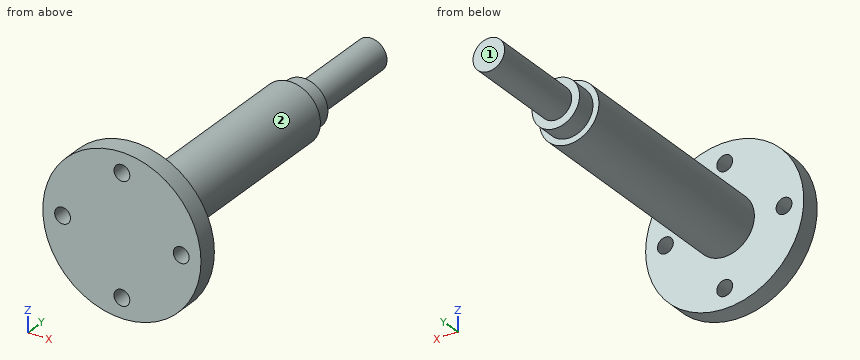
from build123d import *

# Parameters (mm, degrees)
SKETCH1_R           = 20
BOSS_EXTRUDE1_DEPTH = 5
SKETCH2_R           = 7.5
BOSS_EXTRUDE2_DEPTH = 63
SKETCH3_R           = 4
BOSS_EXTRUDE3_DEPTH = 25
SKETCH4_R           = 2
CUT_EXTRUDE1_DEPTH  = 25
SKETCH5_R           = 7.5
SKETCH5_R_2         = 6
CUT_EXTRUDE2_DEPTH  = 5


with BuildPart() as part:
    # Sketch1 → Boss-Extrude1 (new body)
    with BuildSketch(Plane(origin=(0, 0, 0), x_dir=(1, 0, 0), z_dir=(0, 1, 0))):
        Circle(SKETCH1_R)
    extrude(amount=BOSS_EXTRUDE1_DEPTH)

    # Sketch2 → Boss-Extrude2 (add)
    with BuildSketch(Plane(origin=(0, 5, 0), x_dir=(1, 0, 0), z_dir=(0, 1, 0))):
        Circle(SKETCH2_R)
    extrude(amount=BOSS_EXTRUDE2_DEPTH)

    # Sketch3 → Boss-Extrude3 (add)
    with BuildSketch(Plane(origin=(0, 68, 0), x_dir=(1, 0, 0), z_dir=(0, 1, 0))):
        Circle(SKETCH3_R)
    extrude(amount=BOSS_EXTRUDE3_DEPTH)

    # Sketch4 → Cut-Extrude1 (cut)
    with BuildSketch(Plane(origin=(0, 5, 0), x_dir=(1, 0, 0), z_dir=(0, 1, 0))):
        with Locations((0, 15)):
            Circle(SKETCH4_R)
        with Locations((15, 0)):
            Circle(SKETCH4_R)
        with Locations((0, -15)):
            Circle(SKETCH4_R)
        with Locations((-15, 0)):
            Circle(SKETCH4_R)
    extrude(amount=-CUT_EXTRUDE1_DEPTH, mode=Mode.SUBTRACT)

    # Sketch5 → Cut-Extrude2 (cut)
    with BuildSketch(Plane(origin=(0, 68, 0), x_dir=(1, 0, 0), z_dir=(0, 1, 0))):
        Circle(SKETCH5_R)
        Circle(SKETCH5_R_2, mode=Mode.SUBTRACT)
    extrude(amount=-CUT_EXTRUDE2_DEPTH, mode=Mode.SUBTRACT)


solid = part.part
Input: part model. Units: mm. Frame: model coordinates. Face numbers are marked on the shaded views. A direction names the side the tool comes from. Round coordinates to 2 decimals unless told otherwise and drop trailing zeros. Loops run counter-clockwise (first coordinate to the right, second up) from the corner with the lowest first, then second, coordinate; pieces in that order, holes last. Notation, with made-up numbers: (20.5, -28) -> (38.5, -28) arc R36 ccw to (38.5, 8) -> close; hole circle Ø5 at (-20, 60.5). An arc over 180 degrees is marked (long way). Answer as a JSON object with one key per item and string values. Group by question number.
1) Ray query, L1, parallel to X at y = 2.85, z = 0; L2, parallel to Y at x = -7.5, z = -7.5. Return the intervals inside material, ascending.
2) Pin query (flat end, axial travel): pin 1 (3 mm diameter, centred on x = 0, z = -11, fed in from +Y); pin 2 (3 mm diameter, centred on y = 63.5, z = 4, fed in from +X); pin 3 (1.5 mm diameter, centred on x = -1.5, y = 68, fed in from +Z). Return the tip coordinate at first contact, or that it passes through.
3) Section query C-C on z = -15. Output: boundary loops of the cut face in (x, y), plus the area to 3 significant figures.
4) Section query A-A on z = 0. Output: boundary loops of the cut face in (x, y).
5) Section query B-B on x = -15. Output: boundary loops of the cut face in (y, z).
6) Section query D-D on y = 61. Output: boundary loops of the cut face in (x, z).
7) Reachability of the marked faces 1 and 2 from +Z, -Z, +X, -X, +Y, -Y: full face, straight path, thin tool, end or side. Return the list, or none.
Reply:
{
 "1": {"L1": "x = -20 to -17, -13 to 13, 17 to 20", "L2": "y = 0 to 5"},
 "2": {"pin 1": "stops at y = 5", "pin 2": "stops at x = 7.04", "pin 3": "stops at z = 5.95"},
 "3": {"outline": "(-13.23, 0) -> (-2, 0) -> (-2, 5) -> (-13.23, 5) -> close; (2, 0) -> (13.23, 0) -> (13.23, 5) -> (2, 5) -> close", "area": "112 mm2"},
 "4": {"outline": "(-20, 0) -> (-17, 0) -> (-17, 5) -> (-20, 5) -> close; (-13, 0) -> (13, 0) -> (13, 5) -> (7.5, 5) -> (7.5, 63) -> (6, 63) -> (6, 68) -> (4, 68) -> (4, 93) -> (-4, 93) -> (-4, 68) -> (-6, 68) -> (-6, 63) -> (-7.5, 63) -> (-7.5, 5) -> (-13, 5) -> close; (17, 0) -> (20, 0) -> (20, 5) -> (17, 5) -> close"},
 "5": {"outline": "(0, -13.23) -> (5, -13.23) -> (5, -2) -> (0, -2) -> close; (0, 2) -> (5, 2) -> (5, 13.23) -> (0, 13.23) -> close"},
 "6": {"outline": "circle Ø15 at (0, 0)"},
 "7": {"face 1": "+Z, -Z, +X, -X, +Y", "face 2": "+Y"}
}
